```python
from build123d import *

# Parameters (mm, degrees)
SKETCH1_W                     = 120
SKETCH1_H                     = 60
BASE_FLANGE1_DEPTH            = 1.5
BREAK_CORNER1_START           = -1.5
BREAK_CORNER1_DEPTH           = 1.5
CUT_EXTRUDE1_DEPTH            = 10
EDGE_FLANGE3_STRIP_W          = 7.4732
EDGE_FLANGE3_STRIP_H          = 1.5
EDGE_FLANGE3_STRIP_CUT_DEPTH  = 20
EDGE_FLANGE3_RELIEF_W         = 8.9732
EDGE_FLANGE3_RELIEF_H         = 1.5
EDGE_FLANGE3_RELIEF_CUT_DEPTH = 1.5
EDGE_FLANGE3_DEPTH            = 20
MIRROR2_COPY_1_SKETCH_W       = 7.4732
MIRROR2_COPY_1_SKETCH_H       = 1.5
MIRROR2_COPY_1_DEPTH          = 20
MIRROR2_COPY_2_SKETCH_W       = 8.9732
MIRROR2_COPY_2_SKETCH_H       = 1.5
MIRROR2_COPY_2_DEPTH          = 1.5
MIRROR2_COPY_3_DEPTH          = 20
SKETCH14_R                    = 4
CUT_EXTRUDE2_DEPTH            = 91
BREAK_CORNER2_START           = -30
BREAK_CORNER2_DEPTH           = 60


# Read off the part's stored shape, not the designer's step: Break-Corner1, Break-Corner2
# Sheet-metal steps are written as plain solids
with BuildPart() as part:
    # Sketch1 → Base-Flange1 (new body)
    with BuildSketch(Plane(origin=(0, 0, 0), x_dir=(1, 0, 0), z_dir=(0, 1, 0))):
        Rectangle(SKETCH1_W, SKETCH1_H)
    extrude(amount=-BASE_FLANGE1_DEPTH)

    # Break-Corner1 outline → Break-Corner1 (cut)
    with BuildSketch(Plane(origin=(0, 0, 0), x_dir=(1, 0, 0), z_dir=(0, 1, 0)).offset(BREAK_CORNER1_START)):
        with BuildLine():
            ThreePointArc((50, 30), (57.071067812, 27.071067812), (60, 20))
            Line((60, 20), (60, 30))
            Line((60, 30), (50, 30))
        make_face()
        with BuildLine():
            Line((60, -30), (60, -20))
            ThreePointArc((60, -20), (57.071067812, -27.071067812), (50, -30))
            Line((50, -30), (60, -30))
        make_face()
        with BuildLine():
            ThreePointArc((-60, 20), (-57.071067812, 27.071067812), (-50, 30))
            Line((-50, 30), (-60, 30))
            Line((-60, 30), (-60, 20))
        make_face()
        with BuildLine():
            Line((-60, -30), (-50, -30))
            ThreePointArc((-50, -30), (-57.071067812, -27.071067812), (-60, -20))
            Line((-60, -20), (-60, -30))
        make_face()
    extrude(amount=BREAK_CORNER1_DEPTH, mode=Mode.SUBTRACT)

    # Sketch6 → Cut-Extrude1 (cut)
    with BuildSketch(Plane(origin=(0, 0, 0), x_dir=(1, 0, 0), z_dir=(0, 1, 0))):
        with BuildLine():
            Line((-30, 18), (30, 18))
            ThreePointArc((30, 18), (48, 0), (30, -18))
            Line((30, -18), (-30, -18))
            ThreePointArc((-30, -18), (-48, 0), (-30, 18))
        make_face()
    extrude(amount=-CUT_EXTRUDE1_DEPTH, mode=Mode.SUBTRACT)

    # Edge-Flange3 strip (across the edge) → Edge-Flange3 strip cut (cut)
    with BuildSketch(Plane(origin=(-25, -1.5, 30), x_dir=(0, 0, -1), z_dir=(-1, 0, 0))):
        with Locations((-1.5, -0.75)):
            Rectangle(EDGE_FLANGE3_STRIP_W, EDGE_FLANGE3_STRIP_H)
    edge_flange3_strip_cut = extrude(amount=EDGE_FLANGE3_STRIP_CUT_DEPTH, mode=Mode.SUBTRACT)

    # Edge-Flange3 relief (on the sheet) → Edge-Flange3 relief cut (cut)
    with BuildSketch(Plane(origin=(-25, -1.5, 27.7634), x_dir=(0, 0, -1), z_dir=(0, -1, 0))):
        with Locations((-2.9866, 0.75)):
            Rectangle(EDGE_FLANGE3_RELIEF_W, EDGE_FLANGE3_RELIEF_H)
        with Locations((-2.9866, -20.75)):
            Rectangle(EDGE_FLANGE3_RELIEF_W, EDGE_FLANGE3_RELIEF_H)
    edge_flange3_relief_cut = extrude(amount=-EDGE_FLANGE3_RELIEF_CUT_DEPTH, mode=Mode.SUBTRACT)

    # Edge-Flange3 section (across the edge) → Edge-Flange3 (add)
    with BuildSketch(Plane(origin=(-25, -1.5, 30), x_dir=(0, 0, -1), z_dir=(-1, 0, 0))):
        with BuildLine():
            Line((0, 0.7366), (0, 28.5))
            Line((0, 28.5), (1.5, 28.5))
            Line((1.5, 28.5), (1.5, 0.7366))
            ThreePointArc((1.5, 0.7366), (1.715745145, 0.215745145), (2.2366, 0))
            Line((2.2366, 0), (2.2366, -1.5))
            ThreePointArc((2.2366, -1.5), (0.655084973, -0.844915027), (0, 0.7366))
        make_face()
    edge_flange3 = extrude(amount=EDGE_FLANGE3_DEPTH)

    # Mirror1: Edge-Flange3 strip cut, Edge-Flange3 relief cut, Edge-Flange3 across plane
    add(edge_flange3_strip_cut.mirror(Plane(origin=(0, 0, 0), x_dir=(0, 0, 1), z_dir=(1, 0, 0))), mode=Mode.SUBTRACT)
    add(edge_flange3_relief_cut.mirror(Plane(origin=(0, 0, 0), x_dir=(0, 0, 1), z_dir=(1, 0, 0))), mode=Mode.SUBTRACT)
    add(edge_flange3.mirror(Plane(origin=(0, 0, 0), x_dir=(0, 0, 1), z_dir=(1, 0, 0))))

    # Mirror2: Edge-Flange3 strip cut, Edge-Flange3 relief cut, Edge-Flange3 across plane
    add(edge_flange3_strip_cut.mirror(Plane.XY), mode=Mode.SUBTRACT)
    add(edge_flange3_relief_cut.mirror(Plane.XY), mode=Mode.SUBTRACT)
    add(edge_flange3.mirror(Plane.XY))

    # Mirror2 copy 1 sketch → Mirror2 copy 1 (cut)
    with BuildSketch(Plane(origin=(25, -1.5, -30), x_dir=(0, 0, 1), z_dir=(1, 0, 0))):
        with Locations((-1.5, -0.75)):
            Rectangle(MIRROR2_COPY_1_SKETCH_W, MIRROR2_COPY_1_SKETCH_H)
    extrude(amount=MIRROR2_COPY_1_DEPTH, mode=Mode.SUBTRACT)

    # Mirror2 copy 2 sketch → Mirror2 copy 2 (cut)
    with BuildSketch(Plane(origin=(25, -1.5, -27.7634), x_dir=(0, 0, 1), z_dir=(0, -1, 0))):
        with Locations((-2.9866, 0.75)):
            Rectangle(MIRROR2_COPY_2_SKETCH_W, MIRROR2_COPY_2_SKETCH_H)
        with Locations((-2.9866, -20.75)):
            Rectangle(MIRROR2_COPY_2_SKETCH_W, MIRROR2_COPY_2_SKETCH_H)
    extrude(amount=-MIRROR2_COPY_2_DEPTH, mode=Mode.SUBTRACT)

    # Mirror2 copy 3 sketch → Mirror2 copy 3 (add)
    with BuildSketch(Plane(origin=(25, -1.5, -30), x_dir=(0, 0, 1), z_dir=(1, 0, 0))):
        with BuildLine():
            Line((0, 0.7366), (0, 28.5))
            Line((0, 28.5), (1.5, 28.5))
            Line((1.5, 28.5), (1.5, 0.7366))
            ThreePointArc((1.5, 0.7366), (1.715745145, 0.215745145), (2.2366, 0))
            Line((2.2366, 0), (2.2366, -1.5))
            ThreePointArc((2.2366, -1.5), (0.655084973, -0.844915027), (0, 0.7366))
        make_face()
    extrude(amount=MIRROR2_COPY_3_DEPTH)

    # Sketch14 → Cut-Extrude2 (cut, through all)
    with BuildSketch(Plane.XY.offset(30)):
        with Locations((-35, -20)):
            Circle(SKETCH14_R)
        with Locations((35, -20)):
            Circle(SKETCH14_R)
    extrude(amount=-CUT_EXTRUDE2_DEPTH, mode=Mode.SUBTRACT)

    # Break-Corner2 outline → Break-Corner2 (cut)
    with BuildSketch(Plane.XY.offset(BREAK_CORNER2_START)):
        with BuildLine():
            Line((-25, -30), (-25, -25))
            ThreePointArc((-25, -25), (-26.464466094, -28.535533906), (-30, -30))
            Line((-30, -30), (-25, -30))
        make_face()
        with BuildLine():
            Line((-45, -30), (-40, -30))
            ThreePointArc((-40, -30), (-43.535533906, -28.535533906), (-45, -25))
            Line((-45, -25), (-45, -30))
        make_face()
        with BuildLine():
            Line((45, -30), (45, -25))
            ThreePointArc((45, -25), (43.535533906, -28.535533906), (40, -30))
            Line((40, -30), (45, -30))
        make_face()
        with BuildLine():
            Line((25, -30), (30, -30))
            ThreePointArc((30, -30), (26.464466094, -28.535533906), (25, -25))
            Line((25, -25), (25, -30))
        make_face()
    extrude(amount=BREAK_CORNER2_DEPTH, mode=Mode.SUBTRACT)


solid = part.part
```
Could you check a few things on this model? Use its own coordinates, in mm. A direction names the side the tool comes from. Round coordinates to 2 decimals unless told otherwise and drop trailing zeros. Order: outer loops, then holes, each group sorted by start corner. A loop starts at its lowest first (then second) coordinate and runs counter-clockwise, first axis right, second up. Notation, with made-up numbers: M -14,57 L -10,57 A17 cw -10,66 Z; hole C -37.75,74 d6. An arc over 180 degrees is marked long. One line per question, with ' | ' between items. Start each with the question number.
(1) For P1, Ø1.2, axis at x = -24.5, y = -1, coming from the +Z side; P2, Ø3, axis at y = -16.5, z = -28, coming from the +X side; P3, Ø18, axis at x = -15.5, z = 14.5, coming from the -Y side, each with a flat end and sliding along its axis, tell me the tip position at first contact or that it passes through.
(2) Suppose I cut it at D-D on y = -20. Count the separate pieces of the cut face and the enclosed holes in it, then the cut area to 3 significant figures.
(3) Thinking about a two-plate mould opening in Z: for faces 1 (the face through (37, -16, 28.5)), 2 (the face through (-1, 0, -20)), 3 (the face through (-56.99, -0.76, 27.15)), which applies, +Z half, -Z half, draft (parallel to the pull), parting line (faces both ways), or undercut?
(4) Suppose I cut it at B-B on y = -10.5. List the corners of the cut face in (x, z) for me.
(5) For faces 4 (the face through (27, -29, -29)), 5 (the face through (-43, -29, 29)), 6 (the face through (48, -1, 0)), 7 (the face through (37, -16, -28.5)), 8 (the face through (-34.86, -0.64, -29.33)), which set-ups out of +Z, -Z, +X, -X, +Y, -Y let a thin tool reach every point of the face, with its end or its side?
(6) Please list where these lines run through material, in increasing order: line 1 along Z through (x, y) = (-27, -2.5); line 2 along Y through (x, z) = (6.5, -26.5); line 3 along Y through (x, z) = (-35, -29.4).
(7) Suppose I cut it at A-A on x = 7. List the corners of the cut face in (y, z) for me, then the cut area to 3 significant figures.
(8) Suppose I cut it at C-C on z = 0. List the corners of the cut face in (x, y) for me, then the cut area to 3 significant figures.
Geometry results:
1) P1: z = 29.81 | P2: x = 45 | P3: y = -1.5
2) separate pieces: 8 | enclosed holes: 0 | area: 72.0 mm²
3) face 1: undercut | face 2: draft | face 3: +Z half
4) outline: M -45,-30 L -25,-30 L -25,-28.5 L -45,-28.5 Z; M -45,28.5 L -25,28.5 L -25,30 L -45,30 Z; M 25,-30 L 45,-30 L 45,-28.5 L 25,-28.5 Z; M 25,28.5 L 45,28.5 L 45,30 L 25,30 Z
5) face 4: +Z, -Z, -Y | face 5: +Z, -Z, -X, -Y | face 6: +Y, -Y | face 7: +X, -X, -Y | face 8: -Z, +Y
6) line 1: -30 to -28.5, 28.5 to 30 | line 2: -1.5 to 0 | line 3: -30 to -24, -16 to -0.71
7) outline: M -1.5,-30 L 0,-30 L 0,-18 L -1.5,-18 Z; M -1.5,18 L 0,18 L 0,30 L -1.5,30 Z | area: 36.0 mm²
8) outline: M -60,-1.5 L -48,-1.5 L -48,0 L -60,0 Z; M 48,-1.5 L 60,-1.5 L 60,0 L 48,0 Z | area: 36.0 mm²
